Geometry: final body of the model. Coordinates: model frame, mm. A direction names the side the tool comes from. Give positions to 0.01 mm unless a question says otherwise; leave off trailing zeros. Use one line per item in the form item = value. Start each with the question number.
Item 1: Pull-direction query (Y, two-part tool) for faces 3 (the flat face through (0, 0, 0)), 4 (the cylindrical face through (193.77, -2.76, -3.83)), 5 (the flat face through (84, -41, 125)); classes: released by +Y, released by -Y, zero draft, split by the parting line, or undercut.
Item 2: Section query A-A on y = -58. Give the number of separate pieces and of enclosed holes in the cut face, then the cut area to 3 significant figures.
Item 3: Material intervals for line 1 along Z through (x, y) = (86, -2); line 2 along X through (y, z) = (-14, 62.5); line 3 along Z through (x, y) = (47.5, -35), sorted ascending. Write a range as from..to.
Item 4: Contact query for flat-ended pins moving along their axis: P1, Ø2, axis at x = 22, z = 15, coming from the +Y side; P2, Ø3, axis at x = 76.5, z = 32, coming from the +Y side. Output: stop coordinate, or through.
Item 5: Access query for faces 1 (the cylindrical face through (6.633, -20.858, 6.083)), 2 (the flat face through (84, -80, -2)). Directions: +Z, -Z, +X, -X, +Y, -Y. A direction counts if a zero-diameter tool reaches every point of the face in a straight line with its end or side. Return the directions, or none.
from build123d import *

# Parameters (mm, degrees)
BOSS_EXTRUDE1_DEPTH      = 42
SKETCH4_R                = 12.745
CUT_EXTRUDE2_DEPTH       = 231.623535649
SKETCH7_R                = 9
CUT_EXTRUDE4_DEPTH       = 231.513348808
BOSS_EXTRUDE2_DEPTH      = 20
BOSS_EXTRUDE2_DEPTH_BACK = 60
BOSS_EXTRUDE2_START      = -20
SKETCH8_W                = 300
SKETCH8_H                = 250
FILLET1_R                = 10


with BuildPart() as part:
    # Sketch1 → Revolve1 (revolve)
    with BuildSketch(Plane.XY):
        with BuildLine():
            Line((0, -2.75), (0, 0))
            Line((0, 0), (86.4, 0))
            Line((86.4, 0), (86.4, -51.52))
            add(Edge.make_bspline(
                [(0, -2.75), (26.471278047, -40.623393059), (56.78647802, -59.047909877), (86.4, -51.52)],
                knots=[0, 0, 0, 0, 0.721198988, 0.721198988, 0.721198988, 0.721198988], degree=3))
        make_face()
        with BuildLine():
            ThreePointArc((-18.514834727, -5.5), (-18.086269469, -5.596489171), (-17.740408022, -5.867336362))
            add(Edge.make_bspline(
                [(-17.740408022, -5.867336362), (28.13170189, -65.595276468), (86.4, -63.74)],
                knots=[0, 0, 0, 0.824732104, 0.824732104, 0.824732104], degree=2))
            Line((86.4, -63.74), (86.4, -51.52))
            add(Edge.make_bspline(
                [(0, -2.75), (26.471278047, -40.623393059), (56.78647802, -59.047909877), (86.4, -51.52)],
                knots=[0, 0, 0, 0, 0.721198988, 0.721198988, 0.721198988, 0.721198988], degree=3))
            Line((0, -2.75), (0, 0))
            Line((0, 0), (-19.04, 0))
            ThreePointArc((-19.04, 0), (-20.454213562, -0.585786438), (-21.04, -2))
            Line((-21.04, -2), (-21.04, -3.5))
            ThreePointArc((-21.04, -3.5), (-20.454213562, -4.914213562), (-19.04, -5.5))
            Line((-19.04, -5.5), (-18.514834727, -5.5))
        make_face()
    revolve(axis=Axis((86.4, 0, 0), (0, -1, 0)))

    # Sketch3 → Boss-Extrude1 (add)
    with BuildSketch(Plane(origin=(20, 0, 0), x_dir=(0, 0, -1), z_dir=(1, 0, 0))):
        with BuildLine():
            Line((-61.8, 0), (61.8, 0))
            add(Edge.make_bspline(
                [(61.8, 0), (41.99440737, -40.763024165), (0, -42.307560131)],
                knots=[0, 0, 0, 1, 1, 1], degree=2))
            add(Edge.make_bspline(
                [(-61.8, 0), (-41.99440737, -40.763024165), (0, -42.307560131)],
                knots=[0, 0, 0, 1, 1, 1], degree=2))
        make_face()
    extrude(amount=-BOSS_EXTRUDE1_DEPTH)

    # Sketch4 → Cut-Extrude2 (cut, through all)
    with BuildSketch(Plane(origin=(0, 0, 0), x_dir=(1, 0, 0), z_dir=(0, 1, 0))):
        with Locations(Location((86.4, 0, 0), (0, 0, 180))):
            Circle(SKETCH4_R)
    extrude(amount=-CUT_EXTRUDE2_DEPTH, mode=Mode.SUBTRACT)

    # Sketch7 → Cut-Extrude4 (cut, through all)
    with BuildSketch(Plane(origin=(0, 0, 0), x_dir=(1, 0, 0), z_dir=(0, 1, 0))):
        with Locations(Location((0, 0, 0), (0, 0, 180))):
            Circle(SKETCH7_R)
    extrude(amount=-CUT_EXTRUDE4_DEPTH, mode=Mode.SUBTRACT)


with BuildPart() as body_2:
    # Sketch8 → Boss-Extrude2 (new, two sides: drawn at the far end of the back side and taken through both)
    with BuildSketch(Plane(origin=(0, 0, 0), x_dir=(1, 0, 0), z_dir=(0, 1, 0)).offset(BOSS_EXTRUDE2_START - BOSS_EXTRUDE2_DEPTH_BACK)):
        with Locations((86.4, 0)):
            Rectangle(SKETCH8_W, SKETCH8_H)
    extrude(amount=BOSS_EXTRUDE2_DEPTH + BOSS_EXTRUDE2_DEPTH_BACK)

    # Combine1: cut part
    add(part.part, mode=Mode.SUBTRACT)

    # Fillet1
    fillet1_edges = [body_2.edges().sort_by_distance(p)[0] for p in [
        (99.145000004, -63.396409238, 2e-09),
    ]]
    fillet(fillet1_edges, radius=FILLET1_R)


solid = body_2.part
Answer sheet:
q1.face_3 = released by +Y
q1.face_4 = undercut
q1.face_5 = zero draft
q2.separate_pieces = 2
q2.enclosed_holes = 1
q2.area = 71,200 mm2
q3.line_1 = -125..-107.44, -12.74..12.74, 107.44..125
q3.line_2 = -63.6..11.44, 161.36..236.4
q3.line_3 = -125..-66.31, 66.31..125
q4.P1 = -42.63
q4.P2 = -58.95
q5.face_1 = +Y
q5.face_2 = +Z, -Z, +X, -X, -Y
